Geometry: final body of the model. Coordinates: model frame, mm. Face numbers are marked on the shaded views. A direction names the side the tool comes from. Give positions to 0.01 mm unless a question says otherwise; leave off trailing zeros. Write each loop counter-clockwise with the first axis right and the second up, starting at its lowest first coordinate (ties: lowest second). Pieces come first, ordered by that corner, then holes. Notation, with made-up numbers: (-4.5, 68) -> (48.5, 68) arc R19 ccw to (48.5, 84) -> close; hole circle Ø7 at (34, 29.5). An arc over 180 degrees is marked (long way). Answer as a JSON object with one key per item and string values. Group by question number.
(1) Contact query for flat-ended pins moving along their axis: pin 1 Ø8 at (y, z) = (-8.5, 13) entering from +X; pin 2 Ø1.3 at (x, y) = (115.5, 2.5) entering from -Z; pin 3 Ø1.2 at (x, z) = (96.5, 14.5) entering from +Y; pin 4 Ø9 at (x, z) = (16.55, 5.52) entering from -Y. Output: stop coordinate, or through.
(2) Section query B-B on y = -5.5. Output: boundary loops of the cut face in (x, z).
(3) Section query C-C on x = 129. Output: boundary loops of the cut face in (y, z), plus the area to 3 significant figures.
(4) Draft query along X for the marked faces 3, 4, 5 and 6. Return one class per face: +X half, -X half, draft (parallel to the pull), parting line (faces both ways), or undercut.
(5) Section query A-A on x = 16.55. Output: boundary loops of the cut face in (y, z).
(6) Section query D-D on y = 5.25. State how many separate pieces and enclosed holes the cut face has, plus the area to 3 significant figures.
(7) Set-up query: the marked faces 1 and 2. Return all of +Z, -Z, +X, -X, +Y, -Y with unobstructed straight access to the full face (end or side cutting, diameter ignored); none if empty.
(8) Material intervals for probe 1 along Z at (x, y) = (16.55, -9); probe 2 along Y at (x, z) = (166.5, 14.75); probe 3 along Z at (x, y) = (99.5, -1.5), sorted ascending.
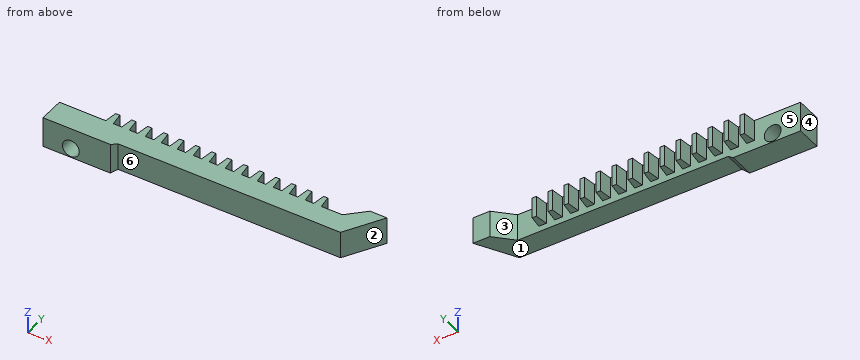
from build123d import *

# Parameters (mm, degrees)
BOSS_EXTRUDE1_DEPTH     = 18
CUT_EXTRUDE3_START      = 10
CUT_EXTRUDE3_DEPTH      = 200.444934928
BOSS_EXTRUDE2_DEPTH     = 12.5
LPATTERN1_COUNT         = 12
LPATTERN1_PITCH         = 9.5
LPATTERN1_COL_COUNT     = 3
LPATTERN1_COL_PITCH     = 9.5
CUT_EXTRUDE2_DEPTH      = 191.497725367
CUT_EXTRUDE2_DEPTH_BACK = 191.497725367
SKETCH5_R               = 5


with BuildPart() as part:
    # Sketch1 → Boss-Extrude1 (new body)
    with BuildSketch(Plane.XY):
        Polygon((0, 0), (167.990381057, 0), (177.990381057, 10), (187.990381057, 10), (175, -12.5), (42.979383981, -12.5), (40, -15), (0, -15), align=None)
    extrude(amount=BOSS_EXTRUDE1_DEPTH)

    # Sketch6 → Cut-Extrude3 (cut, through all)
    with BuildSketch(Plane(origin=(0, 0, 0), x_dir=(1, 0, 0), z_dir=(0, 1, 0)).offset(CUT_EXTRUDE3_START)):
        Polygon((187.990381057, 0), (187.990381057, -2), (42.979383981, -2), (40, 0), align=None)
    extrude(amount=-CUT_EXTRUDE3_DEPTH, mode=Mode.SUBTRACT)

    # Sketch3 → Boss-Extrude2 (add)
    with BuildSketch(Plane.XY.offset(18)):
        Polygon((46.479383981, 0), (50.979383981, 0), (49.979383981, 7.5), (47.479383981, 7.5), align=None)
    boss_extrude2 = extrude(amount=-BOSS_EXTRUDE2_DEPTH)

    # LPattern1: Boss-Extrude2 ×12
    with Locations(*[(i * LPATTERN1_PITCH, 0, 0) for i in range(1, LPATTERN1_COUNT)]):
        add(boss_extrude2)

    # LPattern1 col: Boss-Extrude2 ×3
    with Locations(*[(-i * LPATTERN1_COL_PITCH, 0, 0) for i in range(1, LPATTERN1_COL_COUNT)]):
        add(boss_extrude2)

    # Sketch5 → Cut-Extrude2 (cut, two sides: drawn at the far end of the back side and taken through both)
    with BuildSketch(Plane.XZ.offset(15).offset(-CUT_EXTRUDE2_DEPTH_BACK)):
        with Locations((16.55, 5.52014012)):
            Circle(SKETCH5_R)
    extrude(amount=CUT_EXTRUDE2_DEPTH + CUT_EXTRUDE2_DEPTH_BACK, mode=Mode.SUBTRACT)


solid = part.part
Answer list:
{
 "1": {"pin 1": "x = 179.62", "pin 2": "z = 5.5", "pin 3": "y = 7.5", "pin 4": "through"},
 "2": {"outline": "(0, 0) -> (40, 0) -> (42.98, 2) -> (179.04, 2) -> (179.04, 18) -> (0, 18) -> close; hole circle Ø10 at (16.55, 5.52)"},
 "3": {"outline": "(-12.5, 2) -> (0, 2) -> (0, 18) -> (-12.5, 18) -> close", "area": "200 mm2"},
 "4": {"face 3": "undercut", "face 4": "-X half", "face 5": "undercut", "face 6": "draft"},
 "5": {"outline": "(-15, 0) -> (0, 0) -> (0, 0.52) -> (-15, 0.52) -> close; (-15, 10.52) -> (0, 10.52) -> (0, 18) -> (-15, 18) -> close"},
 "6": {"separate pieces": "15", "enclosed holes": "0", "area": "735 mm2"},
 "7": {"face 1": "-Z, +X, +Y, -Y", "face 2": "+Z, -Z, +X, -Y"},
 "8": {"probe 1": "0 to 0.52, 10.52 to 18", "probe 2": "-12.5 to 0", "probe 3": "2 to 18"}
}
